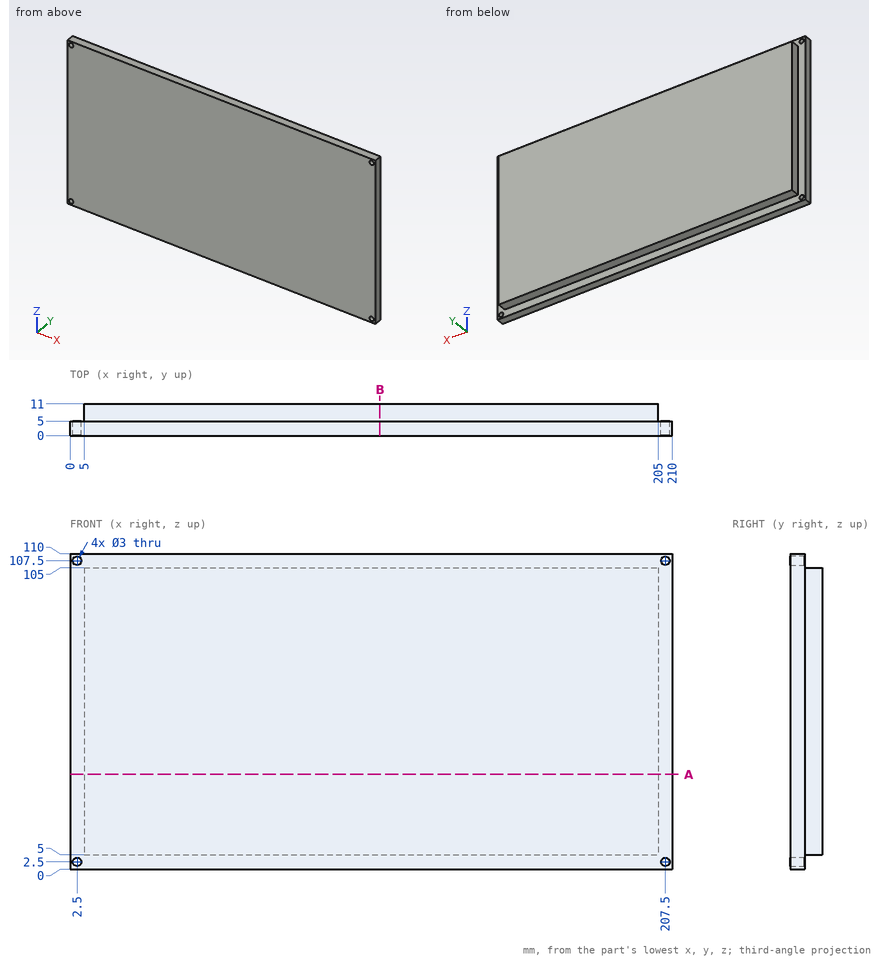
Geometry check sheet. Reference: drawing and pictorial views, mm from the part's lowest x, y, z. Coordinates: 2 decimals unless noted, no trailing zeros. Order: outer loops, then holes, each group sorted by start corner. A loop starts at its lowest first (then second) coordinate and runs counter-clockwise, first axis right, second up. Notation, with made-up numbers: (-5, 38) -> (19, 38) arc R31 cw to (19, 69) -> close; hole circle Ø8 at (-13, 66). An arc over 180 degrees is marked (long way). Write item = value, one per line. Start each with the question number.
1) Cross-section at B-B (x = 108). Enter the section's corners in (y, z), then the cut area to 3 significant figures.
2) Cross-section at A-A (z = 33). Enter the section's corners in (x, y), then the cut area to 3 significant figures.
3) Go/stop test with flat-tipped pins: P1, Ø2.5, axis at x = 2.5, z = 107.5, coming from the -Y side; P2, Ø3, axis at y = 8.5, z = 39, coming from the -X side; P3, Ø5, axis at x = 207.5, z = 2.5, coming from the +Y side; P4, Ø5, axis at y = 8.5, z = 70, coming from the +X side. Record where each tip stops, or that it passes through.
4) Material ranges on L1, parallel to Z at x = 207.5, y = 3.45; L2, parallel to X at y = 2.5, z = 2.5; L3, parallel to Z at x = 80.5, y = 7.75, recorded low to high.
Ans:
q1.outline = (0, 0) -> (5, 0) -> (5, 5) -> (11, 5) -> (11, 105) -> (5, 105) -> (5, 110) -> (0, 110) -> close
q1.area = 1,150 mm²
q2.outline = (0, 0) -> (210, 0) -> (210, 5) -> (205, 5) -> (205, 11) -> (5, 11) -> (5, 5) -> (0, 5) -> close
q2.area = 2,250 mm²
q3.P1 = through
q3.P2 = 5
q3.P3 = 5
q3.P4 = 205
q4.L1 = 0 to 1, 4 to 106, 109 to 110
q4.L2 = 0 to 1, 4 to 206, 209 to 210
q4.L3 = 5 to 105
